from build123d import *

# Parameters (mm, degrees)
SKETCH1_R           = 2.45
SKETCH1_R_2         = 1.625
BOSS_EXTRUDE1_DEPTH = 12
SKETCH1_4_R         = 1.625
BOSS_EXTRUDE2_DEPTH = 3
FILLET1_R           = 0.15


with BuildPart() as part:
    # Sketch1 → Boss-Extrude1 (new body)
    with BuildSketch(Plane(origin=(0, 0, 0), x_dir=(1, 0, 0), z_dir=(0, 1, 0))):
        with Locations(Location((0, 0, 0), (0, 0, 270))):
            Circle(SKETCH1_R)
        with Locations(Location((0, 0, 0), (0, 0, 270))):
            Circle(SKETCH1_R_2, mode=Mode.SUBTRACT)
    extrude(amount=BOSS_EXTRUDE1_DEPTH)

    # Sketch1<4> → Boss-Extrude2 (add)
    with BuildSketch(Plane(origin=(0, 0, 0), x_dir=(1, 0, 0), z_dir=(0, 1, 0))):
        with Locations(Location((0, 0, 0), (0, 0, 270))):
            Circle(SKETCH1_4_R)
    extrude(amount=BOSS_EXTRUDE2_DEPTH)

    # Fillet1
    fillet1_edges = [part.edges().sort_by_distance(p)[0] for p in [
        (0, 12, -2.45),
        (0, 12, -1.625),
    ]]
    fillet(fillet1_edges, radius=FILLET1_R)


solid = part.part
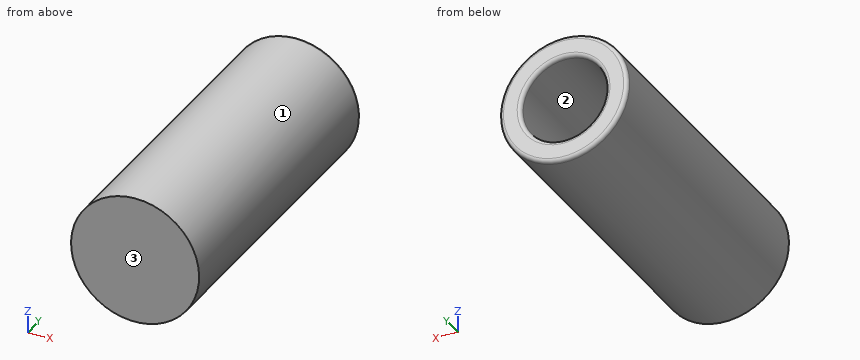
Could you check a few things on this model? Use its own coordinates, in mm. Face numbers are marked on the shaded views. Give positions to 0.01 mm unless a question says otherwise; leave off trailing zeros. Order: outer loops, then holes, each group sorted by start corner. A loop starts at its lowest first (then second) coordinate and runs counter-clockwise, first axis right, second up. Notation, with made-up numbers: (15.5, 89) -> (26.5, 89) arc R14 cw to (26.5, 97) -> close; hole circle Ø1 at (14.5, 33.5). An arc over 180 degrees is marked (long way). Answer in a Markdown table with one row per item. Add a question column.
Item 1: Imagine slicing it at C-C (y = 10.5). List the corners of the cut face in (x, z) for me (3 decimals), and give its area (3 significant figures).
Item 2: We'd pull the mould along X, two halves only. Please class the marked faces 1, 2 and 3: pulls with the +X half, pulls with the -X half, needs draft (parallel to the pull), parting line crosses it, or undercut.
Item 3: Please list where these lines run through material, in increasing order: probe 1 along X at (y, z) = (5.5, 0) (3 decimals); probe 2 along Z at (x, y) = (0.1, 4.25); probe 3 along Z at (x, y) = (0.1, 2.75).
Item 4: Imagine slicing it at B-B (x = 0). List the corners of the cut face in (y, z) for me (3 decimals).
Item 5: Imagine slicing it at A-A (z = 0). List the corners of the cut face in (x, y) for me (3 decimals).
Item 6: I'm going to push flat-ended pins straight in: P1, Ø2.5, axis at x = 0, z = 0, coming from the +Y side; P2, Ø1, axis at x = -1.5, y = 8.5, coming from the +Z side; P3, Ø1.5, axis at y = 2, z = -2, coming from the +X side. Where does each tip first touch, or does it pass through?
Item 7: Imagine slicing it at D-D (y = 2.75). List the corners of the cut face in (x, z) for me.
Result:
| question | item | result |
|---|---|---|
| 1 | outline | circle Ø4.9 at (0, 0); hole circle Ø3.25 at (0, 0) |
| 1 | area | 10.6 mm2 |
| 2 | face 1 | parting line crosses it |
| 2 | face 2 | undercut |
| 2 | face 3 | needs draft |
| 3 | probe 1 | -2.45 to -1.625, 1.625 to 2.45 |
| 3 | probe 2 | -2.45 to -1.62, 1.62 to 2.45 |
| 3 | probe 3 | -2.45 to 2.45 |
| 4 | outline | (0, -2.45) -> (11.85, -2.45) arc R0.15 ccw to (12, -2.3) -> (12, -1.775) arc R0.15 ccw to (11.85, -1.625) -> (3, -1.625) -> (3, 1.625) -> (11.85, 1.625) arc R0.15 ccw to (12, 1.775) -> (12, 2.3) arc R0.15 ccw to (11.85, 2.45) -> (0, 2.45) -> close |
| 5 | outline | (-2.45, 0) -> (2.45, 0) -> (2.45, 11.85) arc R0.15 ccw to (2.3, 12) -> (1.775, 12) arc R0.15 ccw to (1.625, 11.85) -> (1.625, 3) -> (-1.625, 3) -> (-1.625, 11.85) arc R0.15 ccw to (-1.775, 12) -> (-2.3, 12) arc R0.15 ccw to (-2.45, 11.85) -> close |
| 6 | P1 | y = 3 |
| 6 | P2 | z = 2.24 |
| 6 | P3 | x = 2.11 |
| 7 | outline | circle Ø4.9 at (0, 0) |
